Here's how the part is built. I have some questions about the finished solid (model axes, mm). Coordinates: 2 decimals unless noted, no trailing zeros. Write each loop counter-clockwise with the first axis right and the second up, starting at its lowest first coordinate (ties: lowest second). Pieces come first, ordered by that corner, then holes.
(1) Imagine slicing it at A-A, the plane x = -136.5. List the corners of the cut face in (y, z) for me (3 decimals), plus the area to 3 significant figures.
(2) Imagine slicing it at B-B, the plane z = 10.5. List the corners of the cut face in (x, y) for me (3 decimals).
(3) Imagine slicing it at D-D, the plane x = 78. List the corners of the cut face in (y, z) for me (3 decimals), plus the area to 3 significant figures.
(4) Imagine slicing it at C-C, the plane y = -0.9. State how many separate pieces and enclosed holes the cut face has, plus the area to 3 significant figures.
(5) Please list where these lines run through material, in increasing order: probe 1 along Z at (x, y) = (-156, -2.35); probe 2 along Z at (x, y) = (-77.5, -2); probe 3 along X at (y, z) = (-0.2, 27.5).
(6) For pin 1 Ø1.6 at (x, y) = (-112, -1) entering from -Z; pin 2 Ø1 at (y, z) = (-1.5, -46) entering from -X, each with a flat end and sliding along its axis, tell me the tip position at first contact or that it passes through.
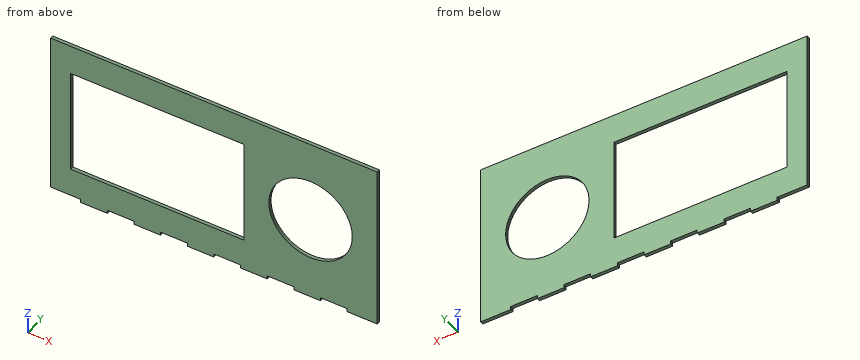
```python
from build123d import *

# Parameters (mm, degrees)
F1_DEPTH = 3.175
F2_W     = 165.1
F2_H     = 100
F2_R     = 39.75
F3_DEPTH = 25.4
F4_W     = 3.175
F4_H     = 25.4
F4_H_2   = 28.575
F4_W_2   = 25.4
F4_H_3   = 3.175
F5_DEPTH = 3.175


# Not quite as in the source:
# - a length typed as a fraction of an inch, garbled in the dataset ("3 / 203.2 mm" for 3/8 in), is restored


with BuildPart() as f1:
    # F0 (on Front) → F1 (new body)
    with BuildSketch(Plane.XZ):
        Polygon((-178.9622853069, -44.2643848114), (-153.5622853069, -44.2643848114), (-153.5622853069, -47.4393848114), (-128.1622853069, -47.4393848114), (-128.1622853069, -44.2643848114), (-102.7622853069, -44.2643848114), (-102.7622853069, -47.4393848114), (-77.3622853069, -47.4393848114), (-77.3622853069, -44.2643848114), (-51.9622853069, -44.2643848114), (-51.9622853069, -47.4393848114), (-26.5622853069, -47.4393848114), (-26.5622853069, -44.2643848114), (-1.1622853069, -44.2643848114), (-1.1622853069, -47.4393848114), (24.2377146931, -47.4393848114), (24.2377146931, -44.2643848114), (49.6377146931, -44.2643848114), (49.6377146931, -47.4393848114), (75.0377146931, -47.4393848114), (75.0377146931, -44.2643848114), (100.4377146931, -44.2643848114), (100.4377146931, -47.4393848114), (125.8377146931, -47.4393848114), (129.0127146931, -47.4393848114), (129.0127146931, -44.2643848114), (129.0127146931, -18.8643848114), (125.8377146931, -18.8643848114), (125.8377146931, 6.5356151886), (129.0127146931, 6.5356151886), (129.0127146931, 31.9356151886), (125.8377146931, 31.9356151886), (125.8377146931, 57.3356151886), (129.0127146931, 57.3356151886), (129.0127146931, 82.7356151886), (125.8377146931, 82.7356151886), (125.8377146931, 108.1356151886), (125.8377146931, 111.3106151886), (100.4377146931, 111.3106151886), (100.4377146931, 108.1356151886), (75.0377146931, 108.1356151886), (75.0377146931, 111.3106151886), (49.6377146931, 111.3106151886), (49.6377146931, 108.1356151886), (24.2377146931, 108.1356151886), (24.2377146931, 111.3106151886), (-1.1622853069, 111.3106151886), (-1.1622853069, 108.1356151886), (-26.5622853069, 108.1356151886), (-26.5622853069, 111.3106151886), (-51.9622853069, 111.3106151886), (-51.9622853069, 108.1356151886), (-77.3622853069, 108.1356151886), (-77.3622853069, 111.3106151886), (-102.7622853069, 111.3106151886), (-102.7622853069, 108.1356151886), (-128.1622853069, 108.1356151886), (-128.1622853069, 111.3106151886), (-153.5622853069, 111.3106151886), (-153.5622853069, 108.1356151886), (-178.9622853069, 108.1356151886), (-178.9622853069, 82.7356151886), (-182.1372853069, 82.7356151886), (-182.1372853069, 57.3356151886), (-178.9622853069, 57.3356151886), (-178.9622853069, 31.9356151886), (-182.1372853069, 31.9356151886), (-182.1372853069, 6.5356151886), (-178.9622853069, 6.5356151886), (-178.9622853069, -18.8643848114), (-182.1372853069, -18.8643848114), (-182.1372853069, -44.2643848114), align=None)
    extrude(amount=F1_DEPTH)

    # F2 (on face) → F3 (cut)
    with BuildSketch(Plane.XZ.offset(3.175)):
        with Locations((-80.5372853069, 33.0406151886)):
            Rectangle(F2_W, F2_H)
        with Locations((65.5127146931, 33.0406151886)):
            Circle(F2_R)
    extrude(amount=-F3_DEPTH, mode=Mode.SUBTRACT)

    # F4 (on face) → F5 (join)
    with BuildSketch(Plane.XZ.offset(3.175)):
        Polygon((-182.1372853069, 111.3106151886), (-182.1372853069, 82.7356151886), (-178.9622853069, 82.7356151886), (-178.9622853069, 108.1356151886), (-153.5622853069, 108.1356151886), (-153.5622853069, 111.3106151886), align=None)
        with Locations((-180.5497853069, 44.6356151886)):
            Rectangle(F4_W, F4_H)
        with Locations((-180.5497853069, -6.1643848114)):
            Rectangle(F4_W, F4_H)
        with Locations((127.4252146931, -6.1643848114)):
            Rectangle(F4_W, F4_H)
        with Locations((127.4252146931, 44.6356151886)):
            Rectangle(F4_W, F4_H)
        with Locations((127.4252146931, 97.0231151886)):
            Rectangle(F4_W, F4_H_2)
        with Locations((87.7377146931, 109.7231151886)):
            Rectangle(F4_W_2, F4_H_3)
        with Locations((36.9377146931, 109.7231151886)):
            Rectangle(F4_W_2, F4_H_3)
        with Locations((-13.8622853069, 109.7231151886)):
            Rectangle(F4_W_2, F4_H_3)
        with Locations((-64.6622853069, 109.7231151886)):
            Rectangle(F4_W_2, F4_H_3)
        with Locations((-115.4622853069, 109.7231151886)):
            Rectangle(F4_W_2, F4_H_3)
    extrude(amount=-F5_DEPTH)


solid = f1.part
```
Recorded:
1. outline: (-3.175, -47.439) - (0, -47.439) - (0, -16.959) - (-3.175, -16.959) - close; (-3.175, 83.041) - (0, 83.041) - (0, 111.311) - (-3.175, 111.311) - close
1. area: 187 mm2
2. outline: (-182.137, -3.175) - (-163.087, -3.175) - (-163.087, 0) - (-182.137, 0) - close; (2.013, -3.175) - (32.772, -3.175) - (32.772, 0) - (2.013, 0) - close; (98.254, -3.175) - (129.013, -3.175) - (129.013, 0) - (98.254, 0) - close
3. outline: (-3.175, -44.264) - (0, -44.264) - (0, -4.697) - (-3.175, -4.697) - close; (-3.175, 70.778) - (0, 70.778) - (0, 111.311) - (-3.175, 111.311) - close
3. area: 254 mm2
4. separate pieces: 1
4. enclosed holes: 2
4. area: 27,400 mm2
5. probe 1: z = -44.26 to -16.96, 83.04 to 111.31
5. probe 2: z = -47.44 to -16.96, 83.04 to 111.31
5. probe 3: x = -182.14 to -163.09, 2.01 to 26.15, 104.87 to 129.01
6. pin 1: stops at z = -44.26
6. pin 2: stops at x = -153.56
